Input: part model. Units: mm. Frame: model coordinates. A direction names the side the tool comes from. Round coordinates to 2 decimals unless told otherwise and drop trailing zeros. Loops run counter-clockwise (first coordinate to the right, second up) from the corner with the lowest first, then second, coordinate; pieces in that order, holes last. Notation, with made-up numbers: M -22,27 L -5,27 A15 cw -5,37 Z; hole C 48.5,57.5 d11. An arc over 180 degrees is marked long. Put each result on its own line as item: value. Start each with the question number.
1) Line query: probe 1 along Z at (x, y) = (9, 39); probe 2 along Y at (x, z) = (10.5, 7); probe 3 along Z at (x, y) = (8, 35.5). Output: solid intervals per line, ascending.
2) Pin query (flat end, axial travel): pin 1 (1.5 mm diameter, centred on x = -9, z = 3, fed in from -Y); pin 2 (13 mm diameter, centred on x = 1, y = -10.5, fed in from -Z); pin 3 (9 mm diameter, centred on x = -5, z = 19.5, fed in from -Y). Return the tip coordinate at first contact, or that it passes through.
3) Section B-B on y = -15.5. Output: boundary loops of the cut face in (x, z), plus the area to 3 significant figures.
4) Section D-D on z = 2. Output: boundary loops of the cut face in (x, y), plus the area to 3 significant figures.
5) Draft query along X for faces 1 (the face through (14.6, 25, 5)), 2 (the face through (0, 4.75, 2)), 3 (the face through (0, 40, 3.2)). Return one class per face: +X half, -X half, draft (parallel to the pull), parting line (faces both ways), or undercut.
6) Section A-A on x = -0.25. Output: boundary loops of the cut face in (y, z).
7) Reachability of faces 4 (the face through (0, 55.45, 25)), 5 (the face through (3.6, -9, 2)), 6 (the face through (-0.2, 51.51, 47.56)), 7 (the face through (-4, -8, 0)), 8 (the face through (-10, -23.25, -1)) from +Z, -Z, +X, -X, +Y, -Y: full face, straight path, thin tool, end or side. Return the list, or none.
8) Section C-C on z = 24. Output: boundary loops of the cut face in (x, y).
from build123d import *

# Parameters (mm, degrees)
PAD002_DEPTH = 5
PAD001_DEPTH = 29.2
FILLET001_R  = 1
PAD_DEPTH    = 3.2
FILLET_R     = 2.2
CHAMFER_SIZE = 2.6


with BuildPart() as body002:
    # Sketch002 (on Face1 of ReferenceFillet) → Pad002 (new body)
    with BuildSketch(Plane(origin=(0, 0, 0), x_dir=(1, 0, 0), z_dir=(0, 0, -1))):
        Polygon((14.6, -55.45), (14.6, 23.25), (8.6, 23.25), (8.6, -9.75), (-8.6, -9.75), (-8.6, 23.25), (-14.6, 23.25), (-14.6, -55.45), align=None)
    extrude(amount=PAD002_DEPTH)


with BuildPart() as body001:
    # Sketch001 (on Face1 of Binder) → Pad001 (new body)
    with BuildSketch(Plane.YZ.offset(14.6)):
        Polygon((23.25, 0), (55.45, 0), (55.45, 56.859816), (52.25, 56.859816), (23.25, 3.2), align=None)
        Polygon((26.660087, 3.2), (52.25, 3.2), (52.25, 50.55), align=None, mode=Mode.SUBTRACT)
    extrude(amount=-PAD001_DEPTH)

    # Fillet001
    fillet001_edges = [body001.edges().sort_by_distance(p)[0] for p in [
        (0, 52.25, 3.2),
        (0, 26.660087, 3.2),
        (0, 52.25, 50.55),
        (0, 52.25, 56.859816),
        (0, 55.45, 56.859816),
    ]]
    fillet(fillet001_edges, radius=FILLET001_R)


with BuildPart() as chamfer_body:
    # Sketch → Pad (new body)
    with BuildSketch(Plane.XY):
        Polygon((-14.6, 23.25), (-14.6, -23.25), (-3.6, -23.25), (-3.6, 4.75), (3.6, 4.75), (3.6, -23.25), (14.6, -23.25), (14.6, 23.25), align=None)
    extrude(amount=PAD_DEPTH)

    # Fillet
    fillet_edges = [chamfer_body.edges().sort_by_distance(p)[0] for p in [
        (9.1, -23.25, 3.2),
        (-9.1, -23.25, 3.2),
    ]]
    fillet(fillet_edges, radius=FILLET_R)

    # Fusion: union Body002, Body001
    add(body002.part)
    add(body001.part)

    # Chamfer
    chamfer_edges = [chamfer_body.edges().sort_by_distance(p)[0] for p in [
        (-8.6, -6.75, 0),
        (0, 9.75, 0),
        (8.6, -6.75, 0),
    ]]
    chamfer(chamfer_edges, length=CHAMFER_SIZE)


solid = chamfer_body.part
Geometry results:
1. probe 1: z = -5 to 3.2, 26.03 to 32.34
1. probe 2: y = 25.3 to 28.71, 52.25 to 55.45
1. probe 3: z = -5 to 3.2, 19.56 to 25.87
2. pin 1: stops at y = -22.86
2. pin 2: stops at z = -1.5
2. pin 3: stops at y = 29.63
3. outline: M -14.6,-5 L -8.6,-5 L -8.6,-2.6 L -6,0 L -3.6,0 L -3.6,3.2 L -14.6,3.2 Z; M 3.6,0 L 6,0 L 8.6,-2.6 L 8.6,-5 L 14.6,-5 L 14.6,3.2 L 3.6,3.2 Z
3. area: 137 mm²
4. outline: M -14.6,-23.01 L -3.6,-23.01 L -3.6,4.75 L 3.6,4.75 L 3.6,-23.01 L 14.6,-23.01 L 14.6,55.45 L -14.6,55.45 Z
4. area: 2,090 mm²
5. face 1: +X half
5. face 2: undercut
5. face 3: draft
6. outline: M 4.75,0 L 7.15,0 L 9.75,-2.6 L 9.75,-5 L 55.45,-5 L 55.45,55.86 A1 ccw 54.45,56.86 L 52.85,56.86 A1 ccw 51.97,56.34 L 23.25,3.2 L 4.75,3.2 Z; hole M 27.46,4.68 A1 ccw 28.34,3.2 L 51.25,3.2 A1 ccw 52.25,4.2 L 52.25,46.6 A1 ccw 50.37,47.07 Z
7. face 4: +Z, -Z, +X, -X, +Y
7. face 5: +Z, -Z, -Y
7. face 6: +X, -X
7. face 7: -Z, -Y
7. face 8: +Z, -Z, +X, -X, -Y
8. outline: M -14.6,34.49 L 14.6,34.49 L 14.6,37.9 L -14.6,37.9 Z; M -14.6,52.25 L 14.6,52.25 L 14.6,55.45 L -14.6,55.45 Z
